Model file for the job. Use its own axes, mm. Face numbers are marked on the shaded views. A direction names the side the tool comes from. Give positions to 0.01 mm unless a question says otherwise; leave off trailing zeros. Write each loop counter-clockwise with the first axis right and the second up, starting at its lowest first coordinate (ties: lowest second). Pieces come first, ordered by that corner, then holes. Notation, with made-up numbers: M -26.75,85.25 L 23.25,85.25 A27 cw 23.25,119.25 Z; hole C -29,22 d5. An arc over 180 degrees is marked long. Answer as a JSON object with one key per item and string values. Group by question number.
```python
from build123d import *

# Parameters (mm, degrees)
SKETCH_1_R                = 65
EXTRUDE_1_DEPTH           = 30
SKETCH_2_R                = 55
CUT_EXTRUDE_1_DEPTH       = 9
SKETCH_3_R                = 45
CUT_EXTRUDE_2_DEPTH       = 8.5
SKETCH_4_R                = 30
CUT_EXTRUDE_3_DEPTH       = 8.5
CUT_EXTRUDE_START         = -5
SKETCH_5_R                = 45
CUT_EXTRUDE_4_DEPTH       = 5
HOLE_WIZARD_1_D           = 4.8
HOLE_WIZARD_1_CBORE_D     = 8
HOLE_WIZARD_1_CBORE_DEPTH = 1
PATTERN_CIRCULAR_1_COUNT  = 16
EXTRUDE_2_DEPTH           = 15
HOLE_WIZARD_2_D           = 7
HOLE_WIZARD_2_CBORE_D     = 11
HOLE_WIZARD_2_CBORE_DEPTH = 6.8
PATTERN_CIRCULAR_2_COUNT  = 6


with BuildPart() as part:
    # Sketch 1 → Extrude 1 (new body)
    with BuildSketch(Plane.XY):
        Circle(SKETCH_1_R)
    extrude(amount=EXTRUDE_1_DEPTH)

    # Sketch 2 → Cut-Extrude 1 (cut)
    with BuildSketch(Plane.XY.offset(30)):
        Circle(SKETCH_2_R)
    extrude(amount=-CUT_EXTRUDE_1_DEPTH, mode=Mode.SUBTRACT)

    # Sketch 3 → Cut-Extrude 2 (cut)
    with BuildSketch(Plane.XY.offset(21)):
        Circle(SKETCH_3_R)
    extrude(amount=-CUT_EXTRUDE_2_DEPTH, mode=Mode.SUBTRACT)

    # Sketch 4 → Cut-Extrude 3 (cut)
    with BuildSketch(Plane.XY.offset(12.5)):
        Circle(SKETCH_4_R)
    extrude(amount=-CUT_EXTRUDE_3_DEPTH, mode=Mode.SUBTRACT)

    # Sketch 5 → Cut-Extrude 4 (cut)
    with BuildSketch(Plane(origin=(0, 0, 0), x_dir=(-1, 0, 0), z_dir=(0, 0, -1)).offset(CUT_EXTRUDE_START)):
        with Locations(Location((0, 0, 0), (0, 0, 180))):
            Circle(SKETCH_5_R)
    extrude(amount=CUT_EXTRUDE_4_DEPTH, mode=Mode.SUBTRACT)

    # Hole Wizard 1 (through all)
    with Locations(Plane(origin=(0, 0, 5), x_dir=(-1, 0, 0), z_dir=(0, 0, -1))):
        with Locations((0, 38.5)):
            hole_wizard_1 = CounterBoreHole(HOLE_WIZARD_1_D / 2, HOLE_WIZARD_1_CBORE_D / 2, HOLE_WIZARD_1_CBORE_DEPTH)

    # Pattern Circular 1: Hole Wizard 1 ×16 about axis
    pattern_circular_1_axis = Axis((0, 0, 0), (0, 0, 1))
    for i in range(1, PATTERN_CIRCULAR_1_COUNT):
        add(hole_wizard_1.rotate(pattern_circular_1_axis, i * 360 / PATTERN_CIRCULAR_1_COUNT), mode=Mode.SUBTRACT)

    # Sketch 9 → Extrude 2 (add)
    with BuildSketch(Plane(origin=(0, 0, 0), x_dir=(-1, 0, 0), z_dir=(0, 0, -1))):
        with BuildLine():
            Line((-6.567411783, 77.422623055), (-9.642643143, 69.086076176))
            ThreePointArc((-9.642643143, 69.086076176), (-12.304478409, 65.141619558), (-16.488038646, 62.874037421))
            ThreePointArc((-16.488038646, 62.874037421), (0, 65), (16.488038646, 62.874037421))
            ThreePointArc((16.488038646, 62.874037421), (12.304478409, 65.141619558), (9.642643143, 69.086076176))
            Line((9.642643143, 69.086076176), (6.567411783, 77.422623055))
            ThreePointArc((6.567411783, 77.422623055), (0, 82), (-6.567411783, 77.422623055))
        make_face()
    extrude_2 = extrude(amount=-EXTRUDE_2_DEPTH)

    # Hole Wizard 2 (through all)
    with Locations(Plane.XY.offset(15)):
        with Locations((0, 75)):
            hole_wizard_2 = CounterBoreHole(HOLE_WIZARD_2_D / 2, HOLE_WIZARD_2_CBORE_D / 2, HOLE_WIZARD_2_CBORE_DEPTH)

    # Pattern Circular 2: Extrude 2, Hole Wizard 2 ×6 about axis
    pattern_circular_2_axis = Axis((0, 0, 0), (0, 0, 1))
    add([extrude_2.rotate(pattern_circular_2_axis, i * 360 / PATTERN_CIRCULAR_2_COUNT) for i in range(1, PATTERN_CIRCULAR_2_COUNT)])
    add([hole_wizard_2.rotate(pattern_circular_2_axis, i * 360 / PATTERN_CIRCULAR_2_COUNT) for i in range(1, PATTERN_CIRCULAR_2_COUNT)], mode=Mode.SUBTRACT)


solid = part.part
```
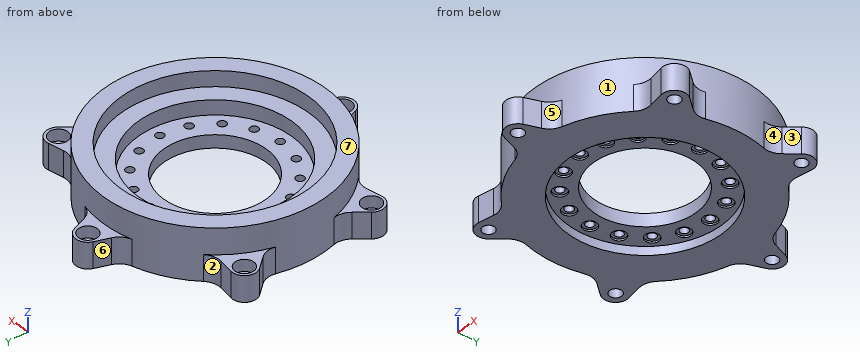
Q1. Wall check: L1, parallel to X at y = 35.5, z = 1.75; L2, parallel to Y at x = 0, z = 10; L3, parallel to Y at x = 0, z = 2. Give the ranges that are in metal, low to high.
Q2. Two-plate mould, pull along Y, no slides. Class the marked faces 4, 5, 6 and 7: +Y half, -Y half, draft (parallel to the pull), parting line (faces both ways), or undercut.
Q3. 3-axis set-ups, long thin cutter, end or side, ignore diameter. For the marked faces 1, 2 and 3: which of +Z, -Z, +X, -X, +Y, -Y reach the whole face in a straight line?
Q4. Slice it at A-A, the plane y = 75. Write the cut outline in (x, z), then the cut area to 3 significant figures.
Q5. Drop flat-ended pins along their axis: P1, Ø9, axis at x = 36, y = 15.5, coming from the -Z side; P2, Ø3, axis at x = 14, y = 49, coming from the +Z side; P3, Ø7, axis at x = 27.22, y = 27.22, coming from the -Z side; P4, Ø7.5, axis at x = -56.5, y = -35.5, coming from the +Z side. Give the stop position or say it passes through.
Q6. Slice it at B-B, the plane y = -47.5. Write the cut outline in (x, z).
Solved:
{
 "1": {"L1": "x = -71.66 to -67.82, -62.08 to -27.65, 27.65 to 62.08, 67.82 to 71.66", "L2": "y = -82 to -80.5, -69.5 to -40.9, -36.1 to -30, 30 to 36.1, 40.9 to 69.5, 80.5 to 82", "L3": "y = -82 to -78.5, -71.5 to -45, 45 to 71.5, 78.5 to 82"},
 "2": {"face 4": "undercut", "face 5": "-Y half", "face 6": "+Y half", "face 7": "draft"},
 "3": {"face 1": "+Z", "face 2": "+Z, -Z, +Y", "face 3": "+Z, -Z, +X"},
 "4": {"outline": "M -7.46,0 L -3.5,0 L -3.5,8.2 L -5.5,8.2 L -5.5,15 L -7.46,15 Z; M 3.5,0 L 7.46,0 L 7.46,15 L 5.5,15 L 5.5,8.2 L 3.5,8.2 Z", "area": "91.6 mm²"},
 "5": {"P1": "stops at z = 5", "P2": "stops at z = 21", "P3": "stops at z = 6", "P4": "stops at z = 30"},
 "6": {"outline": "M -44.37,0 L 44.37,0 L 44.37,30 L 27.73,30 L 27.73,21 L -27.73,21 L -27.73,30 L -44.37,30 Z"}
}
